from build123d import *

# Parameters (mm, degrees)
SKETCH1_W           = 70
SKETCH1_H           = 28
BOSS_EXTRUDE1_DEPTH = 8
SKETCH2_W           = 10
SKETCH2_H           = 10
CUT_EXTRUDE1_DEPTH  = 10
SKETCH3_R           = 2.15
CUT_EXTRUDE2_DEPTH  = 46.530209751
SKETCH5_W           = 16.977623655
SKETCH5_H           = 6.5
CUT_EXTRUDE4_DEPTH  = 39.535697736
FILLET1_R           = 1
CUT_EXTRUDE5_DEPTH  = 10
FILLET2_R           = 2


with BuildPart() as part:
    # Sketch1 → Boss-Extrude1 (new body)
    with BuildSketch(Plane(origin=(0, 0, 0), x_dir=(1, 0, 0), z_dir=(0, 1, 0))):
        Rectangle(SKETCH1_W, SKETCH1_H)
    extrude(amount=BOSS_EXTRUDE1_DEPTH)

    # Sketch2 → Cut-Extrude1 (cut)
    with BuildSketch(Plane(origin=(0, 8, 0), x_dir=(1, 0, 0), z_dir=(0, 1, 0))):
        with Locations((30, 0)):
            Rectangle(SKETCH2_W, SKETCH2_H)
    extrude(amount=-CUT_EXTRUDE1_DEPTH, mode=Mode.SUBTRACT)

    # Sketch3 → Cut-Extrude2 (cut, through all)
    with BuildSketch(Plane.XY.offset(14)):
        with Locations((31, 4)):
            Circle(SKETCH3_R)
    extrude(amount=-CUT_EXTRUDE2_DEPTH, mode=Mode.SUBTRACT)

    # Sketch5 → Cut-Extrude4 (cut, through all)
    with BuildSketch(Plane(origin=(0, 8, 0), x_dir=(1, 0, 0), z_dir=(0, 1, 0))):
        with Locations((-26.511188172, 10.75)):
            Rectangle(SKETCH5_W, SKETCH5_H)
        Polygon((-18.022376345, 14), (-18.022376345, 7.5), (1.977623655, 14), align=None)
        Polygon((1.977623655, -14), (-18.022376345, -7.5), (-18.022376345, -14), align=None)
        with Locations((-26.511188172, -10.75)):
            Rectangle(SKETCH5_W, SKETCH5_H)
    extrude(amount=-CUT_EXTRUDE4_DEPTH, mode=Mode.SUBTRACT)

    # Sketch6 → Cut-Revolve1 (revolve, cut)
    with BuildSketch(Plane.XY):
        with BuildLine():
            Line((-31, 8), (-27.5, 8))
            Line((-27.5, 8), (-27.5, 0))
            Line((-27.5, 0), (-31, 0))
            ThreePointArc((-31, 0), (-32.815072906, 4), (-31, 8))
        make_face()
    revolve(axis=Axis((-27.5, 8, 0), (0, -1, 0)), mode=Mode.SUBTRACT)

    # Fillet1
    fillet1_edges = [part.edges().sort_by_distance(p)[0] for p in [
        (35, 0, -9.5),
        (30, 0, -5),
        (25, 0, 0),
        (30, 0, 5),
        (35, 8, -9.5),
        (30, 8, -5),
        (25, 8, 0),
        (30, 8, 5),
        (18.488811828, 0, 14),
        (-35, 0, 0),
        (-35, 8, 0),
        (18.488811828, 8, 14),
        (35, 8, 9.5),
        (-26.511188172, 0, -7.5),
        (-8.022376345, 0, -10.75),
        (-26.511188172, 8, -7.5),
        (-8.022376345, 8, -10.75),
        (18.488811828, 0, -14),
        (-8.022376345, 8, 10.75),
        (-26.511188172, 8, 7.5),
        (-8.022376345, 0, 10.75),
        (35, 0, 9.5),
        (-26.511188172, 0, 7.5),
        (-24, 0, 0),
        (-24, 8, 0),
        (18.488811828, 8, -14),
    ]]
    fillet(fillet1_edges, radius=FILLET1_R)

    # Sketch7 → Cut-Extrude5 (cut)
    with BuildSketch(Plane(origin=(0, 8, 0), x_dir=(1, 0, 0), z_dir=(0, 1, 0))):
        Polygon((-15.216541459, 0), (8.390933297, -6), (8.390933297, 6), align=None)
    extrude(amount=-CUT_EXTRUDE5_DEPTH, mode=Mode.SUBTRACT)

    # Fillet2
    fillet2_edges = [part.edges().sort_by_distance(p)[0] for p in [
        (-3.412804081, 0, 3),
        (8.390933297, 0, 0),
        (-3.412804081, 0, -3),
        (-15.216541459, 4, 0),
        (8.390933297, 4, -6),
        (8.390933297, 4, 6),
        (-3.412804081, 8, -3),
        (-3.412804081, 8, 3),
        (8.390933297, 8, 0),
    ]]
    fillet(fillet2_edges, radius=FILLET2_R)


solid = part.part
Could you check a few things on this model? Use its own coordinates, in mm. A direction names the side the tool comes from. Give positions to 0.01 mm unless a question says otherwise; leave off trailing zeros. Order: outer loops, then holes, each group sorted by start corner. A loop starts at its lowest first (then second) coordinate and runs counter-clockwise, first axis right, second up. Notation, with made-up numbers: (42.25, 54.25) -> (92.25, 54.25) arc R23 cw to (92.25, 67.25) -> close; hole circle Ø11 at (79, 83). An arc over 180 degrees is marked (long way). Return JSON: item names as keys, results as strings.
1. I need wall thicknesses on line 1 (Y direction, x = 31, z = -8); line 2 (Z direction, x = 32.5, y = 1); line 3 (Z direction, x = -32, y = 3.25). Which ranges of each line are inside material? Lowest first, please. Write a range as from..to.
Answer list:
{"line 1": "y = 0..1.85, 6.15..8", "line 2": "z = -14..-5, 5..14", "line 3": "z = -7.5..-2.73, 2.73..7.5"}
2. For pin 1 Ø2.5 at (x, y) = (31, 4) entering from +Z (3 decimals); pin 2 Ø1 at (x, y) = (-14.5, 6) entering from +Z, each with a flat end and sliding along its axis, tell me the tip position at first contact or that it passes through.
Answer list:
{"pin 1": "passes through", "pin 2": "stops at z = 8.81"}
3. Imagine slicing it at B-B on x = 27.5. List the corners of the cut face in (y, z) for me.
Answer list:
{"outline": "(0, -13) arc R1 ccw to (1, -14) -> (7, -14) arc R1 ccw to (8, -13) -> (8, -6) arc R1 ccw to (7, -5) -> (1, -5) arc R1 ccw to (0, -6) -> close; (0, 6) arc R1 ccw to (1, 5) -> (7, 5) arc R1 ccw to (8, 6) -> (8, 13) arc R1 ccw to (7, 14) -> (1, 14) arc R1 ccw to (0, 13) -> close"}
4. Imagine slicing it at A-A on y = 4. List the corners of the cut face in (x, z) for me, then the cut area to 3 significant figures.
Answer list:
{"outline": "(-35, -7.5) -> (-18.02, -7.5) -> (1.98, -14) -> (28.85, -14) -> (28.85, -5) -> (25, -5) -> (25, 5) -> (28.85, 5) -> (28.85, 14) -> (1.98, 14) -> (-18.02, 7.5) -> (-35, 7.5) -> close; (33.15, -14) -> (35, -14) -> (35, -5) -> (33.15, -5) -> close; (33.15, 5) -> (35, 5) -> (35, 14) -> (33.15, 14) -> close; hole circle Ø10.63 at (-27.5, 0); hole (-7.59, -1.94) -> (5.9, -5.37) arc R2 ccw to (8.39, -3.43) -> (8.39, 3.43) arc R2 ccw to (5.9, 5.37) -> (-7.59, 1.94) arc R2 ccw to start", "area": "1,210 mm2"}
5. Imagine slicing it at C-C on x = -19.5. List the corners of the cut face in (y, z) for me.
Answer list:
{"outline": "(0, -6.5) arc R1 ccw to (1, -7.5) -> (7, -7.5) arc R1 ccw to (8, -6.5) -> (8, 6.5) arc R1 ccw to (7, 7.5) -> (1, 7.5) arc R1 ccw to (0, 6.5) -> close"}
6. On a 3-axis mill with a long thin cutter (end or side, diameter ignored), from which of +Z, -Z, +X, -X, +Y, -Y can I reach the whole of each face in a straight line? I mean faces 1 (the flat face through (-27, 4, 7.5)), 2 (the cylindrical face through (-0.9, 0.57, 4.26)), 3 (the flat face through (28.8, 4.7, -5)), 4 (the flat face through (-0.94, 4.03, 3.63)). Say none if no direction works.
Answer list:
{"face 1": "+Z, -X, +Y, -Y", "face 2": "-Y", "face 3": "+X, +Y, -Y", "face 4": "+Y, -Y"}
7. Thinking about a two-plate mould opening in Z: for faces 5 (the cylindrical face through (-8.146, 7.715, 10.394)), 6 (the cylindrical face through (8.99, 7.43, -0.05)), 7 (the cylindrical face through (-1.09, 7.43, -4.21)), 8 (the flat face through (-35, 4, 0)), which applies, pulls with the +Z half, pulls with the -Z half, needs draft (parallel to the pull), parting line crosses it, or undercut?
Answer list:
{"face 5": "pulls with the +Z half", "face 6": "undercut", "face 7": "undercut", "face 8": "needs draft"}
